```python
from build123d import *

# Parameters (mm, degrees)
SKETCH1_W               = 64
SKETCH1_H               = 64
BOSS_EXTRUDE1_DEPTH     = 64
CUT_EXTRUDE2_DEPTH      = 97.392449486
CUT_EXTRUDE2_DEPTH_BACK = 64
BOSS_EXTRUDE3_DEPTH     = 64
SKETCH10_R              = 11
BOSS_EXTRUDE4_DEPTH     = 13


with BuildPart() as part:
    # Sketch1 → Boss-Extrude1 (new body)
    with BuildSketch(Plane(origin=(0, 0, 0), x_dir=(1, 0, 0), z_dir=(0, 1, 0))):
        with Locations((1.158774373, 32)):
            Rectangle(SKETCH1_W, SKETCH1_H)
    extrude(amount=-BOSS_EXTRUDE1_DEPTH)

    # Sketch4 → Cut-Extrude2 (cut, two sides: drawn at the far end of the back side and taken through both)
    with BuildSketch(Plane(origin=(0, 0, 0), x_dir=(1, 0, 0), z_dir=(0, 1, 0)).offset(-CUT_EXTRUDE2_DEPTH_BACK)):
        Polygon((20.158774373, -173.670400501), (20.158774373, 0), (20.158774373, 51), (-17.841225627, 51), (-17.841225627, 0), (-17.841225627, -173.670400501), (-17.841225627, -521.011201502), (20.158774373, -521.011201502), align=None)
    extrude(amount=CUT_EXTRUDE2_DEPTH + CUT_EXTRUDE2_DEPTH_BACK, mode=Mode.SUBTRACT)

    # Sketch8 → Boss-Extrude3 (add)
    with BuildSketch(Plane(origin=(33.158774373, 0, 0), x_dir=(0, 0, -1), z_dir=(1, 0, 0))):
        Polygon((51, 0), (0, -64), (51, -64), align=None)
    extrude(amount=-BOSS_EXTRUDE3_DEPTH)

    # Sketch10 → Boss-Extrude4 (add)
    # profile 1 of 2: a face of its own
    with BuildSketch(Plane.XZ.offset(64)):
        with BuildLine():
            Line((-30.841225627, 0), (-55.841225627, 0))
            ThreePointArc((-55.841225627, 0), (-87.841225627, -32), (-55.841225627, -64))
            Line((-55.841225627, -64), (-30.841225627, -64))
            Line((-30.841225627, -64), (-30.841225627, 0))
        make_face()
        with Locations(Location((-55.841225627, -32, 0), (0, 0, 270))):
            Circle(SKETCH10_R, mode=Mode.SUBTRACT)
    # profile 2 of 2: a face of its own
    with BuildSketch(Plane.XZ.offset(64)):
        with BuildLine():
            Line((33.158774373, -64), (58.158774373, -64))
            ThreePointArc((58.158774373, -64), (90.158774373, -32), (58.158774373, 0))
            Line((58.158774373, 0), (33.158774373, 0))
            Line((33.158774373, 0), (33.158774373, -64))
        make_face()
        with Locations(Location((58.158774373, -32, 0), (0, 0, 270))):
            Circle(SKETCH10_R, mode=Mode.SUBTRACT)
    extrude(amount=-BOSS_EXTRUDE4_DEPTH)


solid = part.part
```
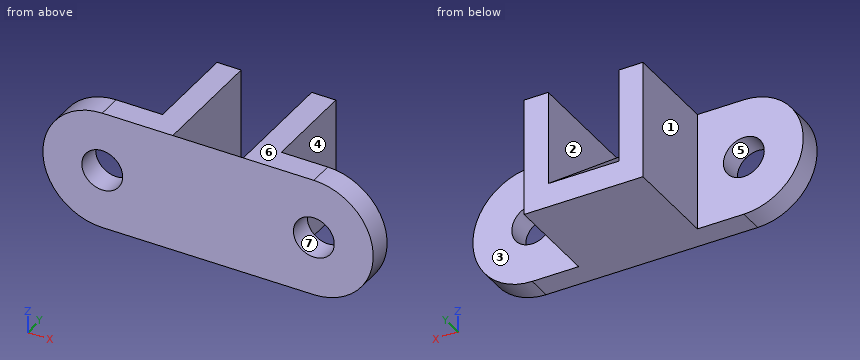
CAD build for the part. Positions are in the model's coordinates, mm. Face numbers are marked on the shaded views. A direction names the side the tool comes from. Coordinates: 2 decimals unless noted, no trailing zeros. Order: outer loops, then holes, each group sorted by start corner. A loop starts at its lowest first (then second) coordinate and runs counter-clockwise, first axis right, second up. Notation, with made-up numbers: M -16,-33.75 L -9,-33.75 A27 ccw -9,-12.75 Z; hole C -6,-9.75 d5. An arc over 180 degrees is marked long. Write each question's results on one line, items separated by ' | '. Start each with the question number.
Q1. Cut at D-D (y = -47.5). List the corners of the cut face in (x, z).
Q2. Pull direction X, two halves, no side cores. Call the marked faces 4, 5, 6 and 7: +X half, -X half, draft (parallel to the pull), parting line (faces both ways), or undercut.
Q3. Drill centre lines: probe 1 along X at (y, z) = (-57, -32); probe 2 along X at (y, z) = (-16.5, -19); probe 3 along X at (y, z) = (-48.5, -51.5). Where is each one in solid material? Low to high. Write a range as from..to.
Q4. Cut at B-B (x = -52). List the corners of the cut face in (y, z), then the cut area to 3 significant figures.
Q5. Flat gauge pins, fed straight in: P1, Ø17, axis at x = 73.5, z = -42.5, coming from the +Y side; P2, Ø15.5, axis at y = -39.5, z = -34, coming from the +X side; P3, Ø2, axis at y = -15.5, z = -31.5, coming from the -X side; P4, Ø2, axis at x = -41.5, y = -48.5, coming from the +Z side. Where does each tip first touch, or does it go through?
Q6. Cut at C-C (y = -57). List the corners of the cut face in (x, z), then the cut area to 3 significant figures.
Q7. Cut at A-A (z = -32). List the corners of the cut face in (x, y).
Q8. Which spindle directions (+Z, -Z, +X, -X, +Y, -Y) get a long thin tool onto all of the face, cutting with end or side? Do the marked faces 1, 2 and 3. Say none if no direction does.
Found:
1) outline: M -30.84,-64 L 33.16,-64 L 33.16,0 L 20.16,0 L 20.16,-13.15 L -17.84,-13.15 L -17.84,0 L -30.84,0 Z
2) face 4: +X half | face 5: undercut | face 6: draft | face 7: undercut
3) probe 1: -87.84..-66.84, -44.84..47.16, 69.16..90.16 | probe 2: -30.84..-17.84, 20.16..33.16 | probe 3: -30.84..33.16
4) outline: M -64,-64 L -51,-64 L -51,-42.31 L -64,-42.31 Z; M -64,-21.69 L -51,-21.69 L -51,0 L -64,0 Z | area: 564 mm²
5) P1: y = -51 | P2: x = 33.16 | P3: x = -30.84 | P4: through
6) outline: M -55.84,-64 L 58.16,-64 A32 ccw 58.16,0 L 20.16,0 L 20.16,-5.58 L -17.84,-5.58 L -17.84,0 L -55.84,0 A32 ccw Z; hole C -55.84,-32 d22; hole C 58.16,-32 d22 | area: 9,540 mm²
7) outline: M -87.84,-64 L -66.84,-64 L -66.84,-51 L -87.84,-51 Z; M -44.84,-64 L 47.16,-64 L 47.16,-51 L 33.16,-51 L 33.16,0 L 20.16,0 L 20.16,-23.84 L -17.84,-23.84 L -17.84,0 L -30.84,0 L -30.84,-51 L -44.84,-51 Z; M 69.16,-64 L 90.16,-64 L 90.16,-51 L 69.16,-51 Z
8) face 1: +Z, -Z, -X, +Y | face 2: +Z, +Y | face 3: +Z, -Z, +X, +Y
